Part print with two shaded views. Sizes in mm from the minimum x, y, z corner. A direction names the side the tool comes from. Give positions to 0.01 mm unless a question says otherwise; leave off trailing zeros. Write each loop counter-clockwise with the first axis right and the second up, starting at its lowest first coordinate (ties: lowest second). Pieces come first, ordered by that corner, then holes. Notation, with made-up numbers: M -7.5,51 L 0.5,51 A23 cw 0.5,76 Z; hole C 89.25,53.25 d1. An arc over 180 degrees is marked long. Return JSON: item names as keys, results as strings. Group by question number.
Q1. Band-saw the part on D-D, the plane x = 3.25. Give the cut face in (y, z), then the cut area to 3 significant figures.
Q2. Band-saw the part on A-A, the plane x = 5. Give the cut face in (y, z).
Q3. Band-saw the part on B-B, the plane y = 4. Give the cut face in (x, z), then the cut area to 3 significant figures.
Q4. Band-saw the part on C-C, the plane z = 7.5. Give the cut face in (x, y), then the cut area to 3 significant figures.
Q5. Flat gauge pins, fed straight in: pin 1 Ø1 at (x, y) = (7.5, 30.5) entering from -Z; pin 2 Ø2.5 at (x, z) = (4.5, 6.5) entering from +Y; pin 3 Ø1 at (x, y) = (7, 7.5) entering from +Z. Where does each tip first touch, or does it go through?
Q6. Wall check: probe 1 along X at (y, z) = (4, 1.1); probe 2 along Y at (x, z) = (5.25, 2.75); probe 3 along Y at (x, z) = (6.25, 8). Give the ranges that are in metal, low to high.
Q7. Tool access for the marked faces 1, 2, 3 and 4: list every direction of +Z, -Z, +X, -X, +Y, -Y with a clear straight run to the whole face (end or side of a thin tool).
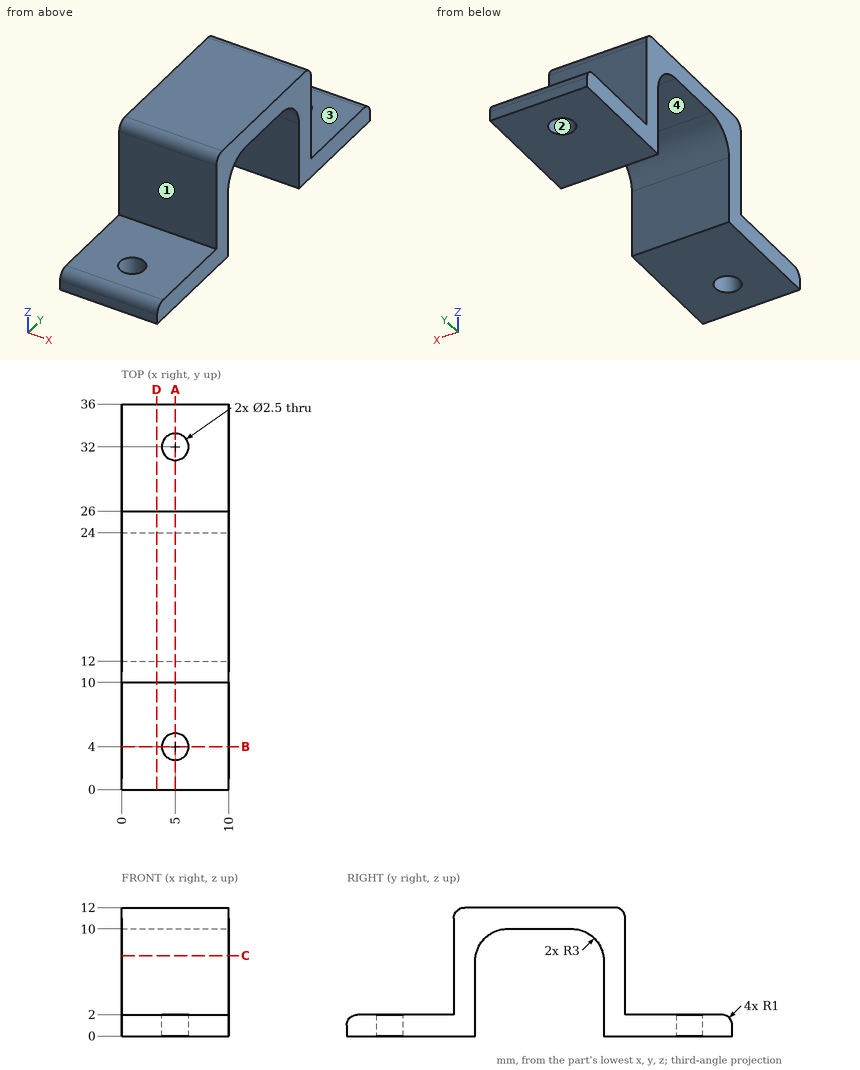
From the geometry:
{
 "1": {"outline": "M 0,0 L 12,0 L 12,7 A3 cw 15,10 L 21,10 A3 cw 24,7 L 24,0 L 36,0 L 36,1 A1 ccw 35,2 L 26,2 L 26,11 A1 ccw 25,12 L 11,12 A1 ccw 10,11 L 10,2 L 1,2 A1 ccw 0,1 Z", "area": "115 mm^2"},
 "2": {"outline": "M 0,0 L 2.75,0 L 2.75,2 L 1,2 A1 ccw 0,1 Z; M 5.25,0 L 12,0 L 12,7 A3 cw 15,10 L 21,10 A3 cw 24,7 L 24,0 L 30.75,0 L 30.75,2 L 26,2 L 26,11 A1 ccw 25,12 L 11,12 A1 ccw 10,11 L 10,2 L 5.25,2 Z; M 33.25,0 L 36,0 L 36,1 A1 ccw 35,2 L 33.25,2 Z"},
 "3": {"outline": "M 0,0 L 3.75,0 L 3.75,2 L 0,2 Z; M 6.25,0 L 10,0 L 10,2 L 6.25,2 Z", "area": "15.0 mm^2"},
 "4": {"outline": "M 0,10 L 10,10 L 10,12.04 L 0,12.04 Z; M 0,23.96 L 10,23.96 L 10,26 L 0,26 Z", "area": "40.8 mm^2"},
 "5": {"pin 1": "stops at z = 0", "pin 2": "stops at y = 26", "pin 3": "stops at z = 2"},
 "6": {"probe 1": "x = 0 to 3.75, 6.25 to 10", "probe 2": "y = 10 to 12, 24 to 26", "probe 3": "y = 10 to 12.17, 23.83 to 26"},
 "7": {"face 1": "+Z, +X, -X, -Y", "face 2": "+Z, -Z", "face 3": "+Z, +X, -X, +Y", "face 4": "-Z, +X, -X"}
}
